Solid Edge part; units mm, degrees
sketch "Sketch1" plane through (0, 0, 0) normal (0, -1, 0) x (1, 0, 0)
  line L0 (132.75, 0) -> (154.75, 0)
  line L1 (154.75, 0) -> (154.75, 10)
  line L2 (154.75, 10) -> (150.75, 10)
  line L3 (150.75, 10) -> (150.75, 4)
  line L4 (150.75, 4) -> (136.75, 4)
  line L5 (136.75, 4) -> (136.75, 10)
  line L6 (136.75, 10) -> (132.75, 10)
  line L7 (132.75, 10) -> (132.75, 0)
  dimension "D1" = 136.75
  dimension "D2" = 154.75
  dimension "D3" = 150.75
  dimension "D4" = 154.75
  dimension "D5" = 132.75
revolve "RevolvedProtrusion1" add sketch "Sketch1" angle 360 about axis through (0, 0, 54) along (0, 0, -1)
properties material "ABS Plastic, high impact"
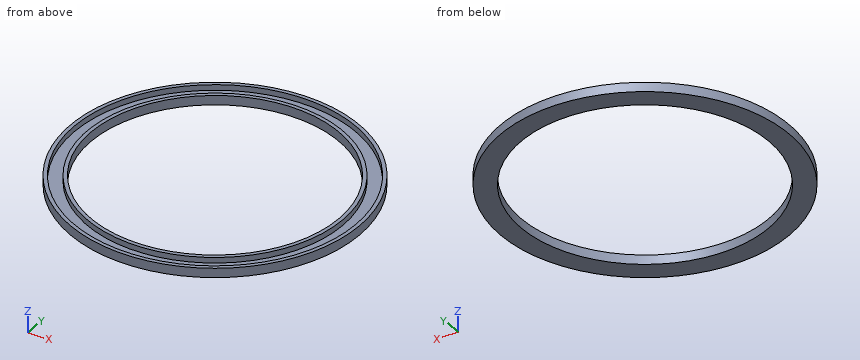
Check sheet for the modelled part. Datum: model origin and axes. Units: mm. Coordinates: 2 decimals unless noted, no trailing zeros. Order: outer loops, then holes, each group sorted by start corner. A loop starts at its lowest first (then second) coordinate and runs counter-clockwise, first axis right, second up. Notation, with made-up numbers: M 21,-22.5 L 71,-22.5 A23 cw 71,4.5 Z; hole C -17.5,73.25 d6. An arc over 180 degrees is marked long. Write each question's results on one line, items separated by ' | '. Start each with the question number.
1. Material ranges on probe 1 along Y at (x, z) = (0, 7.8); probe 2 along X at (y, z) = (0, 2.5), recorded low to high.
2. Cross-section at C-C on z = 7. Record the cut outline in (x, y).
3. Cross-section at A-A on x = 0. Record the cut outline in (y, z), and give its area (3 significant figures).
4. Go/stop test with flat-tipped pins: P1, Ø4, axis at y = 6.5, z = 4.5, coming from the +X side; P2, Ø6, axis at y = 58, z = 6, coming from the -X side; P3, Ø6, axis at x = 36.5, z = 5.5, coming from the +Y side. Record where each tip stops, or that it passes through.
Checks:
1) probe 1: y = -154.75 to -150.75, -136.75 to -132.75, 132.75 to 136.75, 150.75 to 154.75 | probe 2: x = -154.75 to -132.75, 132.75 to 154.75
2) outline: C 0,0 d309.5; C 0,0 d273.5; hole C 0,0 d301.5; hole C 0,0 d265.5
3) outline: M -154.75,0 L -132.75,0 L -132.75,10 L -136.75,10 L -136.75,4 L -150.75,4 L -150.75,10 L -154.75,10 Z; M 132.75,0 L 154.75,0 L 154.75,10 L 150.75,10 L 150.75,4 L 136.75,4 L 136.75,10 L 132.75,10 Z | area: 272 mm²
4) P1: stops at x = 154.68 | P2: stops at x = -144.65 | P3: stops at y = 151.08
